from build123d import *

# Parameters (mm, degrees)
SKETCH1_W               = 246.900926319
SKETCH1_H               = 254
BOSS_EXTRUDE1_DEPTH     = 88.9
SKETCH2_W               = 165.1
SKETCH2_H               = 246.900926319
CUT_EXTRUDE1_DEPTH      = 1
CUT_EXTRUDE1_DEPTH_BACK = 255
SKETCH3_R               = 25.4
BOSS_EXTRUDE2_DEPTH     = 19.05
BOSS_EXTRUDE2_2_DEPTH   = 19.05
BOSS_EXTRUDE2_3_DEPTH   = 19.05
BOSS_EXTRUDE2_4_DEPTH   = 19.05
BOSS_EXTRUDE2_5_DEPTH   = 19.05
BOSS_EXTRUDE3_START     = -82.55
SKETCH4_R               = 6.35
BOSS_EXTRUDE3_DEPTH     = 165.1


with BuildPart() as part:
    # Sketch1 → Boss-Extrude1 (new body, symmetric)
    with BuildSketch(Plane(origin=(0, 0, 0), x_dir=(0, 0, -1), z_dir=(1, 0, 0))):
        with Locations((123.45046316, 127)):
            Rectangle(SKETCH1_W, SKETCH1_H)
    extrude(amount=BOSS_EXTRUDE1_DEPTH, both=True)

    # Sketch2 → Cut-Extrude1 (cut, two sides)
    with BuildSketch(Plane(origin=(0, 254, 0), x_dir=(1, 0, 0), z_dir=(0, 1, 0))) as cut_extrude1_sk:
        with Locations((0, 123.45046316)):
            Rectangle(SKETCH2_W, SKETCH2_H)
    extrude(amount=CUT_EXTRUDE1_DEPTH, mode=Mode.SUBTRACT)
    extrude(cut_extrude1_sk.sketch, amount=-CUT_EXTRUDE1_DEPTH_BACK, mode=Mode.SUBTRACT)



with BuildPart() as body_2:
    # Sketch3 → Boss-Extrude2 (new body, symmetric)
    with BuildSketch(Plane(origin=(0, 0, 0), x_dir=(0, 0, -1), z_dir=(1, 0, 0))):
        with Locations((221.500926319, 215.9)):
            Circle(SKETCH3_R)
    extrude(amount=BOSS_EXTRUDE2_DEPTH, both=True)


with BuildPart() as body_3:
    # Sketch3 → Boss-Extrude2 2 (new body, symmetric)
    with BuildSketch(Plane(origin=(0, 0, 0), x_dir=(0, 0, -1), z_dir=(1, 0, 0))):
        with Locations((25.4, 198.74339204)):
            Circle(SKETCH3_R)
    extrude(amount=BOSS_EXTRUDE2_2_DEPTH, both=True)


with BuildPart() as body_4:
    # Sketch3 → Boss-Extrude2 3 (new body, symmetric)
    with BuildSketch(Plane(origin=(0, 0, 0), x_dir=(0, 0, -1), z_dir=(1, 0, 0))):
        with Locations((221.500926319, 19.05)):
            Circle(SKETCH3_R)
    extrude(amount=BOSS_EXTRUDE2_3_DEPTH, both=True)


with BuildPart() as body_5:
    # Sketch3 → Boss-Extrude2 4 (new body, symmetric)
    with BuildSketch(Plane(origin=(0, 0, 0), x_dir=(0, 0, -1), z_dir=(1, 0, 0))):
        with Locations((123.075926319, 45.422899265)):
            Circle(SKETCH3_R)
    extrude(amount=BOSS_EXTRUDE2_4_DEPTH, both=True)


with BuildPart() as body_6:
    # Sketch3 → Boss-Extrude2 5 (new body, symmetric)
    with BuildSketch(Plane(origin=(0, 0, 0), x_dir=(0, 0, -1), z_dir=(1, 0, 0))):
        with Locations((51.023825584, 117.475)):
            Circle(SKETCH3_R)
    extrude(amount=BOSS_EXTRUDE2_5_DEPTH, both=True)


with BuildPart() as part_1:
    add(part.part)

    add(body_2.part)  # Boss-Extrude3 merges body 2

    add(body_3.part)  # Boss-Extrude3 merges body 3

    add(body_4.part)  # Boss-Extrude3 merges body 4

    add(body_5.part)  # Boss-Extrude3 merges body 5

    add(body_6.part)  # Boss-Extrude3 merges body 6
    # Sketch4 → Boss-Extrude3 (add)
    with BuildSketch(Plane(origin=(0, 0, 0), x_dir=(0, 0, -1), z_dir=(1, 0, 0)).offset(BOSS_EXTRUDE3_START)):
        with Locations((221.500926319, 19.05)):
            Circle(SKETCH4_R)
        with Locations((123.075926319, 45.422899265)):
            Circle(SKETCH4_R)
        with Locations((51.023825584, 117.475)):
            Circle(SKETCH4_R)
        with Locations((25.4, 198.74339204)):
            Circle(SKETCH4_R)
        with Locations((221.500926319, 215.9)):
            Circle(SKETCH4_R)
    extrude(amount=BOSS_EXTRUDE3_DEPTH)


solid = part_1.part
Source: CAD feature listing. Evaluate the final solid. Frame: model axes, mm. A direction names the side the tool comes from. Round coordinates to 2 decimals unless told otherwise and drop trailing zeros. Loops run counter-clockwise (first coordinate to the right, second up) from the corner with the lowest first, then second, coordinate; pieces in that order, holes last.
Q1. Access query for faces 1 (the face through (0.3, 46.5, -97.7)), 2 (the face through (86, 125, -246.901)). Directions: +Z, -Z, +X, -X, +Y, -Y. A direction counts if a zero-diameter tool reaches every point of the face in a straight line with its end or side. Return the directions, or none.
Q2. Mould query, pull axis Y, two halves, no side actions, for faces 3 (the face through (0.27, 173.95, -19.89)), 4 (the face through (-86, 254, -122)), 5 (the face through (19.05, 112, -56)). Classes: pulls with the +Y half, pulls with the -Y half, needs draft (parallel to the pull), parting line crosses it, or undercut.
Q3. Section B-B, the plane y = 215.9. Return loops of the section in (x, z).
Q4. First-contact query: P1, Ø10, axis at x = -7.5, y = 164, coming from the -Z side; P2, Ø1, axis at x = -9, z = -124, coming from the -Y side; P3, Ø3, axis at x = -86, z = -114, coming from the -Y side; P4, Ø12, axis at x = -42.5, y = 116.5, coming from the +Z side. Flat tips, straight axial feed; report the tip coordinate or a pass-through.
Q5. Section C-C, the plane x = -32.5. Return loops of the section in (y, z) (3 decimals).
Q6. Section A-A, the plane z = -181.5. Return loops of the section in (x, y), plus the area to 3 significant figures.
Q7. Ray query, line 1 (X direction, y = 7.5, z = -230); line 2 (X direction, y = 228, z = -56). Return the intervals inside material, ascending.
Solutions:
1. face 1: none
1. face 2: -Z, +X, -X, +Y, -Y
2. face 3: undercut
2. face 4: pulls with the +Y half
2. face 5: needs draft
3. outline: (-88.9, -246.9) - (-82.55, -246.9) - (-82.55, -227.85) - (-19.05, -227.85) - (-19.05, -246.9) - (19.05, -246.9) - (19.05, -227.85) - (82.55, -227.85) - (82.55, -246.9) - (88.9, -246.9) - (88.9, 0) - (82.55, 0) - (82.55, -215.15) - (19.05, -215.15) - (19.05, -196.1) - (-19.05, -196.1) - (-19.05, -215.15) - (-82.55, -215.15) - (-82.55, 0) - (-88.9, 0) - close; (-19.05, -44.13) - (19.05, -44.13) - (19.05, -6.67) - (-19.05, -6.67) - close
4. P1: passes through
4. P2: stops at y = 20.03
4. P3: stops at y = 0
4. P4: stops at z = -44.67
5. outline: circle Ø12.7 at (19.05, -221.501); circle Ø12.7 at (45.423, -123.076); circle Ø12.7 at (117.475, -51.024); circle Ø12.7 at (198.743, -25.4); circle Ø12.7 at (215.9, -221.501)
6. outline: (-88.9, 0) - (-82.55, 0) - (-82.55, 254) - (-88.9, 254) - close; (82.55, 0) - (88.9, 0) - (88.9, 254) - (82.55, 254) - close
6. area: 3,230 mm2
7. line 1: x = -88.9 to -82.55, -19.05 to 19.05, 82.55 to 88.9
7. line 2: x = -88.9 to -82.55, 82.55 to 88.9
